Autodesk Inventor part; units mm, degrees
ref_plane "YZ Plane" through (0, 0, 0) normal (1, 0, 0) x (0, 1, 0)
ref_plane "XZ Plane" through (0, 0, 0) normal (0, 1, 0) x (-1, 0, 0)
ref_plane "XY Plane" through (0, 0, 0) normal (0, 0, 1) x (1, 0, 0)
sketch "Sketch9" plane through (0, 0, 0) normal (0, 0, 1) x (1, 0, 0)
  line L0 (0, 0) -> (0, 55) construction
  circle A0 centre (0, 55) radius 1.5
  circle A1 centre (0, 0) radius 1.5
  circle A2 centre (0, 27.5) radius 1.5
  line L1 (-10, 60) -> (10, 60)
  line L2 (10, 60) -> (10, -5)
  line L3 (10, -5) -> (-10, -5)
  line L4 (-10, -5) -> (-10, 60)
  point P0 (-10, 27.5)
  point P1 (0, 60)
  dimension "d35" = 55
  dimension "d36" = 3
  dimension "d37" = 3
  dimension "d38" = 3
  dimension "d39" = 5
  dimension "d40" = 10
extrude "Extrusion9" add sketch "Sketch9" along normal blind 10
sketch "Sketch11" plane through (10, -5, 0) normal (1, 0, 0) x (0, 0, -1)
  line L0 (0, 65) -> (-10, 65)
  line L1 (0, 65) -> (-75, 65)
  line L2 (-75, 65) -> (-75, 50)
  line L3 (-75, 50) -> (0, 50)
  line L4 (0, 50) -> (0, 65)
  point P0 (0, 5)
  dimension "d43" = 15
  dimension "d44" = 75
extrude "Extrusion10" add sketch "Sketch11" along normal blind 37
sketch "Sketch12" plane through (-10, 60, 10) normal (0, 1, 0) x (1, 0, 0)
  line L0 (20, -65) -> (20, 0)
  line L1 (20, -65) -> (34, -65)
  line L2 (34, -65) -> (34, 0)
  line L3 (34, 0) -> (20, 0)
  line L4 (20, 0) -> (20, -65)
  point P0 (10, 10)
  dimension "d47" = 14
extrude "Extrusion11" cut sketch "Sketch12" against normal through all
chamfer "Chamfer6" distance 14 angle 45 1 edges at (24, 52.5, 10)
sketch "Sketch14" plane through (10, 45, 0) normal (0, -1, 0) x (1, 0, 0)
  line L0 (0, 10) -> (14, 24)
  line L1 (15.4558, 0) -> (37, 21.5442)
  line L2 (37, 75) -> (37, 0)
  line L3 (0, 0) -> (37, 0)
  line L4 (15.4558, 0) -> (37, 0)
  line L5 (37, 21.5442) -> (37, 0)
  point P0 (-10, 0)
  dimension "d73" = 18
extrude "Extrusion13" cut sketch "Sketch14" against normal through all
sketch "Sketch15" plane through (0, 0, 0) normal (0, 0, -1) x (-1, 0, 0)
  line L0 (-25.4558, 60) -> (-25.4558, 45)
  line L1 (-10, 45) -> (-25.4558, 45)
  line L2 (-10, 45) -> (-10, -5)
  line L3 (-10, -5) -> (10, -5)
  line L4 (10, -5) -> (10, 60)
  line L5 (10, 60) -> (-25.4558, 60)
  circle A0 centre (0, 55) radius 1.5
  circle A1 centre (0, 0) radius 1.5
  circle A2 centre (0, 27.5) radius 1.5
  line L6 (-10, -5) -> (10, -5)
  line L7 (10, 60) -> (-10, 60)
  line L8 (-10, -5) -> (-10, 60)
  line L9 (-10, 60) -> (10, 60)
extrude "Extrusion14" add sketch "Sketch15" along normal blind 3 contours L5 L4 L3 L2 L8
chamfer "Chamfer8" distance 3 angle 45 1 edges at (-10, 27.5, 10)
sketch "Sketch17" plane through (-10, -5, -3) normal (0, -1, 0) x (1, 0, 0)
  line L0 (20, 3) -> (20, 13)
  line L1 (20, 3) -> (35.4558, 3)
  line L2 (20, 3) -> (35.4558, 3)
  line L3 (35.4558, 3) -> (37.5981, 4.5)
  line L4 (37.5981, 4.5) -> (51, 4.5)
  line L5 (51, 6.5) -> (36.9675, 6.5)
  line L6 (36.9675, 6.5) -> (34.8252, 5)
  line L7 (34.8252, 5) -> (20, 5)
  line L8 (20, 3) -> (20, 5)
  line L9 (51, 6.5) -> (51, 4.5)
  point P0 (10, 3)
  point P1 (57, 24.5442)
  dimension "d83" = 215
  dimension "d84" = 2
  dimension "d88" = 1.5
  dimension "d89" = 6
extrude "Extrusion16" add sketch "Sketch17" against normal blind 65
sketch "Sketch18" plane through (24, 60, 75) normal (0, 1, 0) x (1, 0, 0)
  line L0 (17, 73.5) -> (3.5981, 73.5)
  line L1 (4.9558, 71.5) -> (17, 71.5)
  line L2 (17, 71.5) -> (17, 73.5)
  line L3 (3.5981, 73.5) -> (4.9558, 71.5)
  point P0 (-24, 75)
extrude "Extrusion17" cut sketch "Sketch18" against normal through all
sketch "Sketch19" plane through (-10, -5, -3) normal (0, -1, 0) x (1, 0, 0)
  line L0 (34.8252, 5) -> (20, 5)
  line L1 (20, 3) -> (35.4558, 3)
  line L2 (35.4558, 3) -> (37.5981, 4.5)
  line L3 (37.5981, 4.5) -> (38.9558, 6.5)
  line L4 (38.9558, 6.5) -> (36.9675, 6.5)
  line L5 (36.9675, 6.5) -> (34.8252, 5)
  line L6 (20, 3) -> (20, 5)
  point P0 (10, 3)
extrude "Extrusion18" cut sketch "Sketch19" against normal blind 50
sketch "Sketch20" plane through (24, 45, 75) normal (0, -1, 0) x (1, 0, 0)
  line L0 (0, 0) -> (0, -51)
  line L1 (-14, -65) -> (0, -51)
  line L2 (1.4558, -75) -> (-14, -75)
  line L3 (-14, -65) -> (-14, -78)
  line L4 (-1, -52) -> (-1, -75)
  line L5 (-14, -75) -> (-1, -75)
  line L6 (-14, -75) -> (-14, -65)
  line L7 (-14, -65) -> (-1, -52)
  line L8 (0, -51) -> (-14, -65)
  point P0 (-24, -75)
  dimension "d94" = 1
extrude "Extrusion19" add sketch "Sketch20" along normal blind 50
chamfer "Chamfer9" distance 5 angle 45 1 edges at (23, 20, 23)
sketch "Sketch21" plane through (24, 45, 75) normal (0, -1, 0) x (1, 0, 0)
  line L0 (-1, -57) -> (-1, -75) construction
  line L1 (1.4558, -75) -> (-1, -75)
  line L2 (3.5981, -73.5) -> (1.4558, -75)
  line L3 (4.9558, -71.5) -> (3.5981, -73.5)
  line L4 (4.9558, -71.5) -> (23, -53.4558)
  line L5 (23, 0) -> (23, -53.4558)
  line L6 (0, 0) -> (23, 0)
  line L7 (0, 0) -> (0, -51)
  line L8 (-4.5355, -55.5355) -> (0, -51)
  line L9 (-1, -57) -> (-4.5355, -55.5355)
  line L10 (4.9558, -71.5) -> (23, -53.4558)
  line L11 (4.9558, -71.5) -> (1.4558, -75)
  line L12 (1.4558, -75) -> (-1, -75)
  point P0 (-24, -75)
extrude "Extrusion20" cut sketch "Sketch21" against normal through all
equation "\"Module\" = 2"
equation "\"PressureAngle\" = 20deg"
equation "\"UnitProfileClearance\" = 0.25"
equation "\"UnitRoundRadius\" = 0.35"
equation "\"HeadDiameter\" = 42"
equation "\"RootDiameter\" = 33"
equation "\"BaseDiameter\" = 35.70832"
equation "\"PitchDiameter\" = 38"
equation "\"HelixAngle\" = 0"
equation "\"UnitCorrection\" = 0"
equation "\"UnitAddendumModification\" = 0"
equation "\"CircularPitch\" = 6.283185"
equation "\"UnitBacklashShift\" = 0"
equation "\"TotalToolShift\" = 0"
equation "\"IsInternal\" = 0"
properties part number "GA04" material "ABS Plastic"
Geometry check sheet. Reference: the model listing, model coordinates, mm. A direction names the side the tool comes from. Coordinates: 2 decimals unless noted, no trailing zeros. Order: outer loops, then holes, each group sorted by start corner. A loop starts at its lowest first (then second) coordinate and runs counter-clockwise, first axis right, second up. Notation, with made-up numbers: M 11,54.25 L 67,54.25 A16 cw 67,83.25 Z; hole C 43.5,40 d2. An arc over 180 degrees is marked long. Use CSV: the item, a comma, the result in double quotes.
Item 1: Thickness scan on line 1 along Y through (x, z) = (0, -1.4); line 2 along X through (y, z) = (0, -2); line 3 along X through (y, z) = (27.5, 5). Record the ranges inside material, lowest first.
Returned:
line 1,"y = -5 to -1.5, 1.5 to 26, 29 to 53.5, 56.5 to 60"
line 2,"x = -10 to -1.5, 1.5 to 10"
line 3,"x = -10 to -1.5, 1.5 to 23"
Item 2: Cross-section at C-C on z = 69. Record the cut outline in (x, y).
Returned:
outline,"M 24,45 L 47,45 L 47,60 L 24,60 Z"
Item 3: Cross-section at B-B on x = 0. Record the cut outline in (y, z), then the cut area to 3 significant figures.
Returned:
outline,"M -5,-3 L -1.5,-3 L -1.5,10 L -5,10 Z; M 1.5,-3 L 26,-3 L 26,10 L 1.5,10 Z; M 29,-3 L 53.5,-3 L 53.5,10 L 29,10 Z; M 56.5,-3 L 60,-3 L 60,10 L 56.5,10 Z"
area,"728 mm2"
Item 4: Cross-section at A-A on y = 27.5. Record the cut outline in (x, z), then the cut area to 3 significant figures.
Returned:
outline,"M -10,-3 L -1.5,-3 L -1.5,10 L -7,10 L -10,7 Z; M 1.5,-3 L 10,-3 L 10,0 L 23,0 L 23,18 L 19.46,19.46 L 10,10 L 1.5,10 Z"
area,"422 mm2"
Item 5: Gauge pin test, flat ends, axial feed: pin 1 Ø8.5 at (x, y) = (1, 18.5) entering from +Z; pin 2 Ø6 at (x, y) = (17, 17.5) entering from -Z; pin 3 Ø12 at (y, z) = (51.5, 47) entering from -X. Record the tip position at first contact, or that the pin passes through.
Returned:
pin 1,"stops at z = 10"
pin 2,"stops at z = 0"
pin 3,"stops at x = 24"
Item 6: Cross-section at D-D on y = 55. Record the cut outline in (x, z).
Returned:
outline,"M -10,-3 L -1.5,-3 L -1.5,10 L -7,10 L -10,7 Z; M 1.5,-3 L 10,-3 L 10,0 L 25.46,0 L 47,21.54 L 47,75 L 24,75 L 24,24 L 10,10 L 1.5,10 Z"
Item 7: Tool access check on faces 1 (the flat face through (2, 28, 10)), 2 (the flat face through (18, 28, 0)), 3 (the flat face through (21.26, 20.35, 18.72)). Record the directions out of +Z, -Z, +X, -X, +Y, -Y that give a thin tool (end or side, any length) a straight path to the whole face; none if there is none.
Returned:
face 1,"+Z, -X, +Y, -Y"
face 2,"-Z, +X, +Y, -Y"
face 3,"+Z, +X, -Y"
